Check sheet for the modelled part. Datum: model origin and axes. Units: mm. Face numbers are marked on the shaded views. Give positions to 0.01 mm unless a question says otherwise; leave off trailing zeros. Order: outer loops, then holes, each group sorted by start corner. A loop starts at its lowest first (then second) coordinate and runs counter-clockwise, first axis right, second up. Notation, with made-up numbers: M -25,-28 L 2,-28 A14 ccw 2,-23 Z; hole C -28.75,79.5 d6. An arc over 180 degrees is marked long. Return JSON: item names as keys, results as strings. Group by question number.
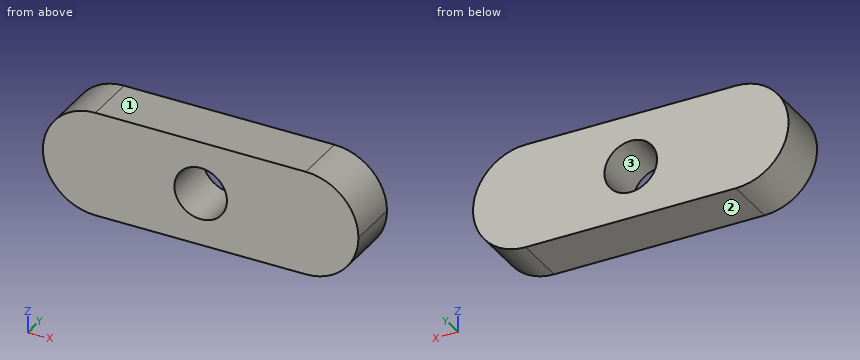
from build123d import *

# Parameters (mm, degrees)
F0_R     = 6.35
F1_DEPTH = 6.35


with BuildPart() as f1:
    # F0 (on Front) → F1 (new body, symmetric)
    with BuildSketch(Plane.XZ):
        with BuildLine():
            Line((25.4, 12.7), (-25.4, 12.7))
            ThreePointArc((-25.4, 12.7), (-16.419744, 8.980256), (-12.7, 0))
            ThreePointArc((-12.7, 0), (-16.419744, -8.980256), (-25.4, -12.7))
            Line((-25.4, -12.7), (25.4, -12.7))
            ThreePointArc((25.4, -12.7), (12.7, 0), (25.4, 12.7))
        make_face()
        Circle(F0_R, mode=Mode.SUBTRACT)
        with BuildLine():
            ThreePointArc((38.1, 0), (34.380256, 8.980256), (25.4, 12.7))
            ThreePointArc((25.4, 12.7), (12.7, 0), (25.4, -12.7))
            ThreePointArc((25.4, -12.7), (34.380256, -8.980256), (38.1, 0))
        make_face()
        with BuildLine():
            ThreePointArc((-12.7, 0), (-16.419744, 8.980256), (-25.4, 12.7))
            ThreePointArc((-25.4, 12.7), (-38.1, 0), (-25.4, -12.7))
            ThreePointArc((-25.4, -12.7), (-16.419744, -8.980256), (-12.7, 0))
        make_face()
    extrude(amount=F1_DEPTH, both=True)


solid = f1.part
1) Sectioned sample at A-A on x = 0. Record the boundary of the cut face in (y, z).
2) Sectioned sample at C-C on y = -3. Record the boundary of the cut face in (x, z).
3) Release check for a two-part mould opening along Z. For the marked faces 1, 2 and 3 record: released by +Z, released by -Z, zero draft, split by the parting line, or undercut.
4) Depth check by flat-ended pin: P1, Ø6, axis at y = -2, z = -4.5, coming from the -X side; P2, Ø6, axis at y = -0.5, z = -6.5, coming from the +X side. Enter the tip coordinate at first touch or a pass-through.
5) Sectioned sample at D-D on z = 10.75. Record the boundary of the cut face in (x, y).
6) Sectioned sample at B-B on z = 1.75. Record the boundary of the cut face in (x, y).
7) Material ranges on line 1 along Z through (x, y) = (0, 3.5); line 2 along X through (y, z) = (-2.75, 1.75); line 3 along X through (y, z) = (6, -2.5), recorded low to high.
Reply:
{
 "1": {"outline": "M -6.35,-12.7 L 6.35,-12.7 L 6.35,-6.35 L -6.35,-6.35 Z; M -6.35,6.35 L 6.35,6.35 L 6.35,12.7 L -6.35,12.7 Z"},
 "2": {"outline": "M -25.4,-12.7 L 25.4,-12.7 A12.7 ccw 25.4,12.7 L -25.4,12.7 A12.7 ccw Z; hole C 0,0 d12.7"},
 "3": {"face 1": "released by +Z", "face 2": "released by -Z", "face 3": "undercut"},
 "4": {"P1": "x = -38.01", "P2": "x = 37.61"},
 "5": {"outline": "M -32.16,-6.35 L 32.16,-6.35 L 32.16,6.35 L -32.16,6.35 Z"},
 "6": {"outline": "M -37.98,-6.35 L -6.1,-6.35 L -6.1,6.35 L -37.98,6.35 Z; M 6.1,-6.35 L 37.98,-6.35 L 37.98,6.35 L 6.1,6.35 Z"},
 "7": {"line 1": "-12.7 to -6.35, 6.35 to 12.7", "line 2": "-37.98 to -6.1, 6.1 to 37.98", "line 3": "-37.85 to -5.84, 5.84 to 37.85"}
}
